Autodesk Inventor part; units mm, degrees
ref_plane "YZ Plane" through (0, 0, 0) normal (1, 0, 0) x (0, 1, 0)
ref_plane "XZ Plane" through (0, 0, 0) normal (0, 1, 0) x (-1, 0, 0)
ref_plane "XY Plane" through (0, 0, 0) normal (0, 0, 1) x (1, 0, 0)
sketch "Sketch1" plane through (0, 0, 0) normal (0, 0, 1) x (1, 0, 0)
  line L0 (199, 195.1016) -> (-199, 195.1016)
  line L1 (-199, 195.1016) -> (-199, -130.8984)
  line L2 (-199, -130.8984) -> (199, -130.8984)
  line L3 (199, -130.8984) -> (199, 195.1016)
  line L4 (-264.1156, 220.8859) -> (-264.1156, -220.8859)
  line L5 (-264.1156, -220.8859) -> (264.1156, -220.8859)
  line L6 (264.1156, -220.8859) -> (264.1156, 220.8859)
  line L7 (264.1156, 220.8859) -> (-264.1156, 220.8859)
  line L8 (-200, 196.1016) -> (200, 196.1016)
  line L9 (200, 196.1016) -> (200, -131.8984)
  line L10 (200, -131.8984) -> (-200, -131.8984)
  line L11 (-200, -131.8984) -> (-200, 196.1016)
  point P0 (0, 0)
  dimension "d0" = 1
extrude "Extrusion1" add sketch "Sketch1" along normal blind 12 contours L7 L6 L5 L4
sketch "Sketch2" plane through (0, 0, 0) normal (0, 0, -1) x (-1, 0, 0)
  point P0 (0, 0)
  point P1 (-219.1094, -175.8797)
  point P2 (219.1094, -175.8797)
hole "Hole1" at (219.1094, -175.8797, 0) at (-219.1094, -175.8797, 0) direction (0, 0, 1) diameter 23 end through all
sketch "Sketch3" plane through (0, 0, 0) normal (0, 0, -1) x (-1, 0, 0)
  circle A0 centre (-202.5, 180.5016) radius 3
  circle A1 centre (-202.5, 172.0016) radius 2
  line L0 (199, 195.1016) -> (-199, 195.1016)
  circle A2 centre (-129, 198.6016) radius 2
  circle A3 centre (0, 198.6016) radius 2
  circle A4 centre (129, 198.6016) radius 2
  circle A5 centre (202.5, 180.5016) radius 3
  circle A6 centre (202.5, 172.0016) radius 2
  line L1 (199, -130.8984) -> (199, 195.1016)
  circle A7 centre (202.5, 32.1016) radius 2
  line L2 (199, -130.8984) -> (199, 195.1016)
  circle A8 centre (202.5, -107.7984) radius 2
  circle A9 centre (202.5, -116.2984) radius 3
  circle A10 centre (-202.5, -116.2984) radius 3
  circle A11 centre (-202.5, -107.7984) radius 2
  circle A12 centre (-202.5, 32.1016) radius 2
  point P0 (0, 0)
hole "Hole2" at (202.5, 180.5016, 0) at (202.5, 172.0016, 0) at (129, 198.6016, 0) at (0, 198.6016, 0) at (-129, 198.6016, 0) at (-202.5, 180.5016, 0) at (-202.5, 172.0016, 0) at (202.5, 32.1016, 0) at (202.5, -116.2984, 0) at (202.5, -107.7984, 0) at (-202.5, -116.2984, 0) at (-202.5, 32.1016, 0) at (-202.5, -107.7984, 0) direction (0, 0, 1) diameter 2.5 end through all
properties part number "lag2"
Work out the finished part from the listing and answer in its coordinate system (mm). A direction names the side the tool comes from. Round coordinates to 2 decimals unless told otherwise and drop trailing zeros. Write each loop counter-clockwise with the first axis right and the second up, starting at its lowest first coordinate (ties: lowest second). Pieces come first, ordered by that corner, then holes.
1) A cutting plane is placed at A-A on x = 36.5. Determine the outline of the cut face in (y, z), and give its area (3 significant figures).
2) A cutting plane is placed at D-D on y = -171. Determine the outline of the cut face in (x, z).
3) Which of the six approach directions +Z, -Z, +X, -X, +Y, -Y give full straight-line access (tool end or side, diameter ignored) to faces 1 (the face through (4, 220.886, 6)), 2 (the face through (200, 34, 6))?
4) Determine the mould class of faces 3 (the face through (264.116, -3, 6)), 4 (the face through (-264.116, 3, 6)), 5 (the face through (209.41, -169.7, 6.08)) for opening direction X: pulls with the +X half, pulls with the -X half, needs draft (parallel to the pull), parting line crosses it, or undercut.
5) Consider probe 1 along Y at (x, z) = (-202.5, 3); probe 2 along Y at (x, z) = (-102.5, 9.75); probe 3 along X at (y, z) = (134, 3.25). Determine where each line is inside the solid, lowest interval first.
6) Flat-ended cylindrical pins translate along their axes: P1, Ø4, axis at x = -202.5, y = -107.8, coming from the -Z side; P2, Ø1.5, axis at x = -202.5, y = 172, coming from the -Z side. Find the tip coordinate at first contact, or state that the pin passes through.
7) A cutting plane is placed at B-B on y = -78. Determine the outline of the cut face in (x, z).
8) A cutting plane is placed at C-C on z = 4.25. Give the number of separate pieces and of enclosed holes in the cut face, and give its area (3 significant figures).
Entries:
1. outline: (-220.89, 0) - (-131.9, 0) - (-131.9, 12) - (-220.89, 12) - close; (196.1, 0) - (220.89, 0) - (220.89, 12) - (196.1, 12) - close
1. area: 1,370 mm2
2. outline: (-264.12, 0) - (-229.52, 0) - (-229.52, 12) - (-264.12, 12) - close; (-208.7, 0) - (208.7, 0) - (208.7, 12) - (-208.7, 12) - close; (229.52, 0) - (264.12, 0) - (264.12, 12) - (229.52, 12) - close
3. face 1: +Z, -Z, +X, -X, +Y
3. face 2: +Z, -Z
4. face 3: pulls with the +X half
4. face 4: pulls with the -X half
4. face 5: undercut
5. probe 1: y = -220.89 to -117.55, -115.05 to -109.05, -106.55 to 30.85, 33.35 to 170.75, 173.25 to 179.25, 181.75 to 220.89
5. probe 2: y = -220.89 to -131.9, 196.1 to 220.89
5. probe 3: x = -264.12 to -200, 200 to 264.12
6. P1: stops at z = 0
6. P2: passes through
7. outline: (-264.12, 0) - (-200, 0) - (-200, 12) - (-264.12, 12) - close; (200, 0) - (264.12, 0) - (264.12, 12) - (200, 12) - close
8. separate pieces: 1
8. enclosed holes: 16
8. area: 101,000 mm2
